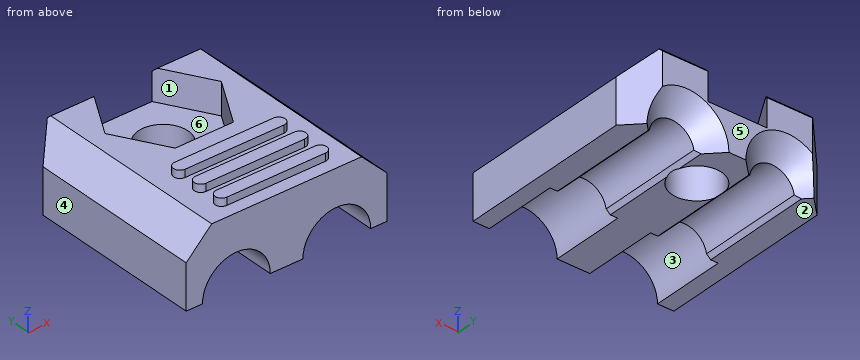
Autodesk Inventor part; units mm, degrees
ref_plane "YZ Plane" through (0, 0, 0) normal (1, 0, 0) x (0, 1, 0)
ref_plane "XZ Plane" through (0, 0, 0) normal (0, 1, 0) x (-1, 0, 0)
ref_plane "XY Plane" through (0, 0, 0) normal (0, 0, 1) x (1, 0, 0)
sketch "Sketch1" plane through (0, 0, 0) normal (0, 1, 0) x (-1, 0, 0)
  line L0 (-10.2591, 9.049) -> (9.7409, 9.049)
  line L1 (9.7409, 9.049) -> (9.7409, -10.951)
  line L2 (9.7409, -10.951) -> (-10.2591, -10.951)
  line L3 (-10.2591, -10.951) -> (-10.2591, 9.049)
  point P0 (0, 0)
  dimension "d0" = 20
  dimension "d1" = 20
extrude "Extrusion1" add sketch "Sketch1" along normal blind 7
sketch "Sketch2" plane through (-9.7409, 0, 9.049) normal (0, 0, 1) x (1, 0, 0)
  line L0 (20, 0) -> (0, 0)
  line L1 (20, 0) -> (20, 7)
  line L2 (0, 0) -> (0, 7)
  circle A0 centre (15, 0) radius 3.375
  circle A1 centre (5, 0) radius 3.375
  point P0 (9.7409, 0)
  dimension "d4" = 6.75
  dimension "d5" = 6.75
  dimension "d6" = 5
  dimension "d7" = 5
  dimension "d32" = 10
extrude "Extrusion2" cut sketch "Sketch2" against normal blind 7.4
sketch "Sketch3" plane through (-9.7409, 0, 1.649) normal (0, 0, 1) x (1, 0, 0)
  arc A0 (8.375, 0) -> (1.625, 0) centre (5, 0) ccw
  line L0 (18.375, 0) -> (11.625, 0)
  arc A1 (18.375, 0) -> (11.625, 0) centre (15, 0) ccw
  circle A2 centre (15, 0) radius 2.25
  circle A3 centre (5, 0) radius 2.25
  point P0 (9.7409, 0)
  dimension "d10" = 4.5
  dimension "d11" = 4.5
extrude "Extrusion3" cut sketch "Sketch3" against normal through all contours A2 L0 | L0 A2 | A3
sketch "Sketch4" plane through (0, 0, 0) normal (0, -1, 0) x (1, 0, 0)
  line L0 (-2.4909, 1.649) -> (-2.4909, -10.951)
  line L1 (3.0091, -10.951) -> (3.0091, 1.649)
  circle A0 centre (0.2591, -6.0003) radius 2.4765
  point P0 (0, 0)
  dimension "d14" = 4.953
  dimension "d15" = 5.5
  dimension "d16" = 2.75
extrude "Extrusion4" cut sketch "Sketch4" against normal through all
chamfer "Chamfer1" distance 1.905 angle 45 2 edges at (5.2591, 2.25, -10.951) (-4.7409, 2.25, -10.951)
chamfer "Chamfer2" distance 0.381 angle 45 5 edges at (-2.4909, 0, -3.6985) (-6.9909, 0, -3.6985) (7.5091, 0, -3.6985) (3.0091, 0, -3.6985) (0.2591, 7, -10.951)
chamfer "Chamfer3" distance 2.54 angle 45 4 edges at (-9.7409, 7, -0.7605) (10.2591, 7, -0.7605) (-9.7409, 3.3095, -10.951) (10.2591, 3.3095, -10.951)
sketch "Sketch5" plane through (0, 7, 0) normal (0, 1, 0) x (1, 0, 0)
  line L0 (-7.2009, 10.57) -> (7.7191, 10.57)
  circle A0 centre (0.2591, 6.0003) radius 2.4765
  line L1 (3.1554, 0.9838) -> (-2.6371, 0.9838)
  line L2 (-2.6371, 0.9838) -> (-5.5334, 6.0003)
  line L3 (-5.5334, 6.0003) -> (-2.6371, 11.0168)
  line L4 (-2.6371, 11.0168) -> (3.1554, 11.0168)
  line L5 (3.1554, 11.0168) -> (6.0517, 6.0003)
  line L6 (6.0517, 6.0003) -> (3.1554, 0.9838)
  point P0 (0, 0)
  dimension "d29" = 10.033
extrude "Extrusion5" cut sketch "Sketch5" against normal blind 3.175
sketch "Sketch6" plane through (0, 7, 0) normal (0, 1, 0) x (1, 0, 0)
  line L0 (-7.2009, -9.049) -> (-7.2009, 10.57)
  line L1 (-7.2009, -9.049) -> (7.7191, -9.049)
  line L2 (7.7191, 10.57) -> (7.7191, -9.049)
  line L3 (3.4133, 10.57) -> (7.7191, 10.57)
  line L4 (-4.6609, -7.144) -> (5.1791, -7.144) construction
  line L5 (-4.6609, -7.779) -> (5.1791, -7.779)
  line L6 (5.1791, -6.509) -> (-4.6609, -6.509)
  arc A0 (-4.6609, -6.509) -> (-4.6609, -7.779) centre (-4.6609, -7.144) ccw
  arc A1 (5.1791, -7.779) -> (5.1791, -6.509) centre (5.1791, -7.144) ccw
  line L7 (-4.6609, -5.239) -> (5.1791, -5.239)
  line L8 (5.1791, -3.969) -> (-4.6609, -3.969)
  arc A2 (-4.6609, -3.969) -> (-4.6609, -5.239) centre (-4.6609, -4.604) ccw
  arc A3 (5.1791, -5.239) -> (5.1791, -3.969) centre (5.1791, -4.604) ccw
  line L9 (-4.6609, -2.699) -> (5.1791, -2.699)
  line L10 (5.1791, -1.429) -> (-4.6609, -1.429)
  arc A4 (-4.6609, -1.429) -> (-4.6609, -2.699) centre (-4.6609, -2.064) ccw
  arc A5 (5.1791, -2.699) -> (5.1791, -1.429) centre (5.1791, -2.064) ccw
  point P0 (0, 0)
  point P1 (0.2591, -7.144)
  dimension "d33" = 1.27
  dimension "d34" = 2.54
  dimension "d35" = 2.54
  dimension "d36" = 1.905
  dimension "d39" = 2.54
extrude "Extrusion6" add sketch "Sketch6" along normal blind 0.762
move or copy body "Move Body1" bodies to move or copy 1 copy no rotation origin (0, 0, 0) rotation axis (1, 0, 0) rotation angle 90
equation "\"d16\" = 0.5 * d15"
properties part number "key_half"
For this review, take the finished solid that the model builds, in its own axes (mm). Face numbers are marked on the shaded views. A direction names the side the tool comes from. Round coordinates to 2 decimals unless told otherwise and drop trailing zeros. Loops run counter-clockwise (first coordinate to the right, second up) from the corner with the lowest first, then second, coordinate; pieces in that order, holes last. Notation, with made-up numbers: (64.5, -3.75) - (120.5, -3.75) arc R22 cw to (120.5, 22.25) - close; hole circle Ø7 at (6, 27). An arc over 180 degrees is marked (long way). Answer as CSV lines item,"result".
(1) Tool access review of the marked faces 1, 2 and 3: name each direction out of +Z, -Z, +X, -X, +Y, -Y from which nothing blocks a thin tool from reaching the whole face with its end or side.
Checked values:
face 1,"+Z"
face 2,"-Z, +X, -X, +Y, -Y"
face 3,"-Z, -Y"
(2) Insertion check: P1, Ø3, axis at x = -2, y = 4, coming from the +Z side (3 decimals); P2, Ø0.8, axis at x = 0.5, z = 7.5, coming from the +Y side; P3, Ø1, axis at x = -7.5, y = -1, coming from the +Z side; P4, Ø1, axis at x = -4.5, z = 1, coming from the -Y side. Each pin has a flat end and moves straight along its axis. Give the tip position at first contact, or say it passes through.
Checked values:
P1,"stops at z = 3.825"
P2,"stops at y = -1.43"
P3,"stops at z = 7"
P4,"passes through"
(3) Mouldability with a two-part tool opening along X and no side actions: class the marked faces 4, 5 and 6 as +X half, -X half, draft (parallel to the pull), parting line (faces both ways), or undercut.
Checked values:
face 4,"-X half"
face 5,"draft"
face 6,"undercut"
(4) Consider section C-C on y = 4.75. Give the boundary of the cut face in (x, z) (3 decimals).
Checked values:
outline,"(-9.741, 0) - (-7.372, 0) - (-6.959, 0.38) arc R2.25 cw to (-2.523, 0.38) - (-2.11, 0) - (-1.879, 0) - (-1.879, 3.825) - (-4.812, 3.825) - (-4.812, 7) - (-7.201, 7) - (-9.741, 4.46) - close; (2.397, 0) - (2.628, 0) - (3.041, 0.38) arc R2.25 cw to (7.477, 0.38) - (7.89, 0) - (10.259, 0) - (10.259, 4.46) - (7.719, 7) - (5.33, 7) - (5.33, 3.825) - (2.397, 3.825) - close"
(5) Wall thickness on line 1 (X direction, y = -5.5, z = 2.75); line 2 (X direction, y = -1, z = 1); line 3 (X direction, y = 4.25, z = 1.25): over which ranges is each line inside the solid? List them lowest first.
Checked values:
line 1,"x = -9.74 to -6.7, -2.78 to 3.3, 7.22 to 10.26"
line 2,"x = -9.74 to -6.76, -2.73 to 3.24, 7.27 to 10.26"
line 3,"x = -9.74 to -6.61, -2.87 to -1.49, 2.01 to 3.39, 7.13 to 10.26"
(6) Consider section B-B on x = 0.5. Give the boundary of the cut face in (y, z) (3 decimals), then the cut area to 3 significant figures.
Checked values:
outline,"(-9.049, 0) - (3.536, 0) - (3.536, 3.825) - (0.984, 3.825) - (0.984, 7) - (-1.429, 7) - (-1.429, 7.762) - (-2.699, 7.762) - (-2.699, 7) - (-3.969, 7) - (-3.969, 7.762) - (-5.239, 7.762) - (-5.239, 7) - (-6.509, 7) - (-6.509, 7.762) - (-7.779, 7.762) - (-7.779, 7) - (-9.049, 7) - close; (8.465, 0) - (10.951, 0) - (10.951, 3.825) - (8.465, 3.825) - close"
area,"92.4 mm2"
(7) Consider section D-D on y = 0.5. Give the boundary of the cut face in (x, z), then the cut area to 3 significant figures.
Checked values:
outline,"(-9.74, 0) - (-7.37, 0) - (-6.96, 0.38) arc R2.25 cw to (-2.52, 0.38) - (-2.11, 0) - (2.63, 0) - (3.04, 0.38) arc R2.25 cw to (7.48, 0.38) - (7.89, 0) - (10.26, 0) - (10.26, 4.46) - (7.72, 7) - (-7.2, 7) - (-9.74, 4.46) - close"
area,"117 mm2"
(8) Consider section A-A on z = 7.25. Give the boundary of the cut face in (x, y) (3 decimals), then the cut area to 3 significant figures.
Checked values:
outline,"(-4.661, -7.779) - (5.179, -7.779) arc R0.635 ccw to (5.179, -6.509) - (-4.661, -6.509) arc R0.635 ccw to start; (-4.661, -5.239) - (5.179, -5.239) arc R0.635 ccw to (5.179, -3.969) - (-4.661, -3.969) arc R0.635 ccw to start; (-4.661, -2.699) - (5.179, -2.699) arc R0.635 ccw to (5.179, -1.429) - (-4.661, -1.429) arc R0.635 ccw to start"
area,"41.3 mm2"
